Could you check a few things on this model? Use its own coordinates, in mm. Face numbers are marked on the shaded views. A direction names the side the tool comes from. Coordinates: 2 decimals unless noted, no trailing zeros. Write each loop counter-clockwise with the first axis right and the second up, starting at its lowest first coordinate (ties: lowest second). Pieces come first, ordered by that corner, then holes.
```python
from build123d import *

# Parameters (mm, degrees)
F0_W     = 600
F0_H     = 1200
F1_DEPTH = 500
F2_T     = -50
F3_W     = 50
F3_H     = 100
F4_DEPTH = 300


with BuildPart() as f1:
    # F0 (on Top) → F1 (new body, symmetric)
    with BuildSketch(Plane.XY):
        Rectangle(F0_W, F0_H)
    extrude(amount=F1_DEPTH, both=True)

    # F2
    f2_openings = [f1.faces().sort_by_distance(p)[0] for p in [
        (0, 0, 500),
    ]]
    offset(amount=F2_T, openings=f2_openings)

    # F3 (on Right) → F4 (join, symmetric)
    with BuildSketch(Plane.YZ):
        with Locations((-384.018666, -550)):
            Rectangle(F3_W, F3_H)
        with Locations((384.018666, -550)):
            Rectangle(F3_W, F3_H)
    extrude(amount=F4_DEPTH, both=True)


solid = f1.part
```
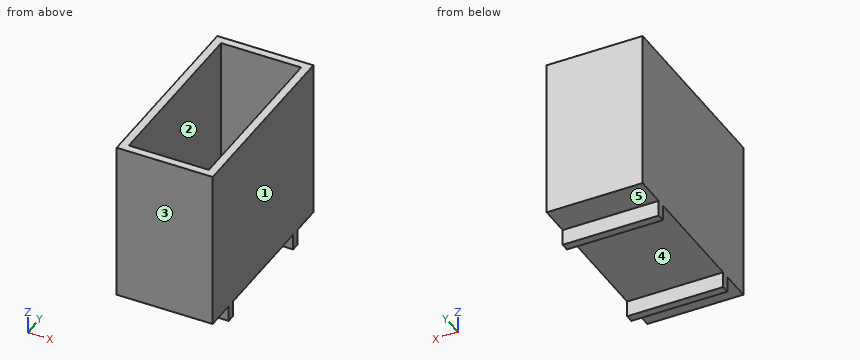
Item 1: If we mould it in two halves opening along Y, with no side actions, what happens to the marked faces 3, 4 and 5? For each: released by +Y, released by -Y, zero draft, split by the parting line, or undercut.
Item 2: I want a section at A-A, the plane z = -81.5. List the corners of the cut face in (x, y) for me.
Item 3: I want a section at D-D, the plane y = 320. List the corners of the cut face in (x, z) for me.
Item 4: Which directions (+Z, -Z, +X, -X, +Y, -Y) give clear straight access to the entire face, cutting with the end or side of a thin tool? Please do the marked faces 1 and 2.
Item 5: Will these pins go through, and if not, where does the flat tip stop? pin 1 Ø5 at (x, y) = (-21.5, -220.5) entering from +Z; pin 2 Ø1 at (x, y) = (156, -148) entering from -Z.
Item 6: I want a section at C-C, the plane y = -388. List the corners of the cut face in (x, z) for me, then the cut area to 3 significant figures.
Item 7: I want a section at B-B, the plane x = 197. List the corners of the cut face in (y, z) for me, then the cut area to 3 significant figures.
Item 8: If I drill on line 1 along Y through (x, z) = (-8.5, -266); line 2 along X through (y, z) = (-6.5, 441); line 3 along Z through (x, y) = (199, 132), over which ranges is the centre line in solid material (lowest first)?
Taken from the geometry:
1. face 3: released by -Y
1. face 4: undercut
1. face 5: zero draft
2. outline: (-300, -600) - (300, -600) - (300, 600) - (-300, 600) - close; hole (-250, -550) - (250, -550) - (250, 550) - (-250, 550) - close
3. outline: (-300, -500) - (300, -500) - (300, 500) - (250, 500) - (250, -450) - (-250, -450) - (-250, 500) - (-300, 500) - close
4. face 1: +Z, -Z, +X, +Y, -Y
4. face 2: +Z
5. pin 1: stops at z = -450
5. pin 2: stops at z = -500
6. outline: (-300, -600) - (300, -600) - (300, 500) - (250, 500) - (250, -450) - (-250, -450) - (-250, 500) - (-300, 500) - close
6. area: 185,000 mm2
7. outline: (-600, -500) - (-409.02, -500) - (-409.02, -600) - (-359.02, -600) - (-359.02, -500) - (359.02, -500) - (359.02, -600) - (409.02, -600) - (409.02, -500) - (600, -500) - (600, 500) - (550, 500) - (550, -450) - (-550, -450) - (-550, 500) - (-600, 500) - close
7. area: 165,000 mm2
8. line 1: y = -600 to -550, 550 to 600
8. line 2: x = -300 to -250, 250 to 300
8. line 3: z = -500 to -450
